Input: part model. Units: mm. Frame: model coordinates. Face numbers are marked on the shaded views. A direction names the side the tool comes from. Give positions to 0.01 mm unless a question says otherwise; leave off trailing zeros. Loops run counter-clockwise (first coordinate to the right, second up) from the corner with the lowest first, then second, coordinate; pieces in that order, holes last.
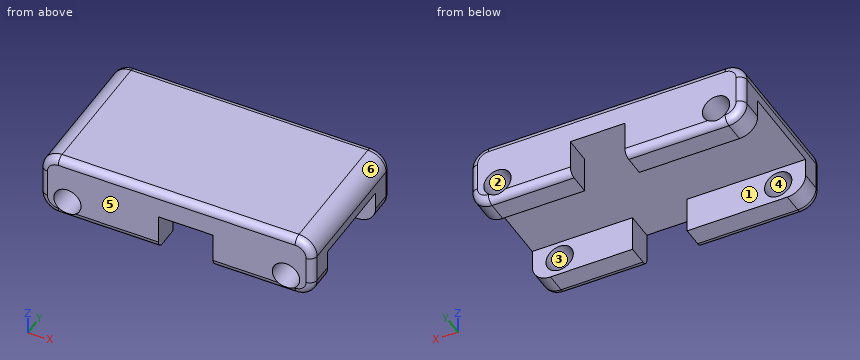
from build123d import *

# Parameters (mm, degrees)
F0_R          = 4.7625
F1_DEPTH      = 25.4
F2_W          = 31.75
F2_H          = 12.7
F3_DEPTH      = 47.626
F3_DEPTH_BACK = 47.626
F4_T1_DEPTH   = 82.55
F4_T3_DEPTH   = 9.6279704779
F4_T5_DEPTH   = 41.275
F4_T7_DEPTH   = 34.925
F4_T10_ANGLE  = 90
F4_T12_ANGLE  = 90
F4_T14_ANGLE  = 90
F4_T16_ANGLE  = 90
F4_T18_ANGLE  = 90
F4_T20_ANGLE  = 90
F4_T22_ANGLE  = 90
F4_T24_ANGLE  = 90


# Not quite as in the source:
# - a fillet or chamfer that OpenCascade refuses, or shapes differently, is made with other operations: its cross-section is extruded or revolved along the edge and cut away or added


with BuildPart() as f1:
    # F0 (on Front) → F1 (new body, symmetric)
    with BuildSketch(Plane.XZ):
        with BuildLine():
            Line((41.275, 15.9779704779), (-41.275, 15.9779704779))
            ThreePointArc((-41.275, 15.9779704779), (-45.7651280605, 14.1180985385), (-47.625, 9.6279704779))
            Line((-47.625, 9.6279704779), (-47.625, 0))
            ThreePointArc((-47.625, 0), (-45.7651280605, -4.4901280605), (-41.275, -6.35))
            Line((-41.275, -6.35), (-6.35, -6.35))
            Line((-6.35, -6.35), (-6.35, 6.35))
            Line((-6.35, 6.35), (12.7, 6.35))
            Line((12.7, 6.35), (12.7, -6.35))
            Line((12.7, -6.35), (41.275, -6.35))
            ThreePointArc((41.275, -6.35), (45.7651280605, -4.4901280605), (47.625, 0))
            Line((47.625, 0), (47.625, 9.6279704779))
            ThreePointArc((47.625, 9.6279704779), (45.7651280605, 14.1180985385), (41.275, 15.9779704779))
        make_face()
        with Locations((-38.1, 0)):
            Circle(F0_R, mode=Mode.SUBTRACT)
        with Locations((38.1, 0)):
            Circle(F0_R, mode=Mode.SUBTRACT)
    extrude(amount=F1_DEPTH, both=True)

    # F2 (on Right) → F3 (cut, two sides)
    with BuildSketch(Plane.YZ) as f3_sk:
        Rectangle(F2_W, F2_H)
    extrude(amount=F3_DEPTH, mode=Mode.SUBTRACT)
    extrude(f3_sk.sketch, amount=-F3_DEPTH_BACK, mode=Mode.SUBTRACT)

    # F4: fillet of radius 2.54 on 18 edges, made by hand

    # F4_s2 → F4_t1 (cut)
    with BuildSketch(Plane.YZ.offset(-41.275)):
        with BuildLine():
            ThreePointArc((22.86, 15.9779704779), (24.6560512242, 15.2340217022), (25.4, 13.4379704779))
            Line((25.4, 13.4379704779), (25.4, 15.9779704779))
            Line((25.4, 15.9779704779), (22.86, 15.9779704779))
        make_face()
        with BuildLine():
            ThreePointArc((-22.86, 15.9779704779), (-24.6560512242, 15.2340217022), (-25.4, 13.4379704779))
            Line((-25.4, 13.4379704779), (-25.4, 15.9779704779))
            Line((-25.4, 15.9779704779), (-22.86, 15.9779704779))
        make_face()
    extrude(amount=F4_T1_DEPTH, mode=Mode.SUBTRACT)

    # F4_s4 → F4_t3 (cut)
    with BuildSketch(Plane.XY):
        with BuildLine():
            ThreePointArc((-45.085, 25.4), (-46.8810512242, 24.6560512242), (-47.625, 22.86))
            Line((-47.625, 22.86), (-47.625, 25.4))
            Line((-47.625, 25.4), (-45.085, 25.4))
        make_face()
        with BuildLine():
            ThreePointArc((45.085, 25.4), (46.8810512242, 24.6560512242), (47.625, 22.86))
            Line((47.625, 22.86), (47.625, 25.4))
            Line((47.625, 25.4), (45.085, 25.4))
        make_face()
        with BuildLine():
            ThreePointArc((-45.085, -25.4), (-46.8810512242, -24.6560512242), (-47.625, -22.86))
            Line((-47.625, -22.86), (-47.625, -25.4))
            Line((-47.625, -25.4), (-45.085, -25.4))
        make_face()
        with BuildLine():
            ThreePointArc((45.085, -25.4), (46.8810512242, -24.6560512242), (47.625, -22.86))
            Line((47.625, -22.86), (47.625, -25.4))
            Line((47.625, -25.4), (45.085, -25.4))
        make_face()
    extrude(amount=F4_T3_DEPTH, mode=Mode.SUBTRACT)

    # F4_s6 → F4_t5 (cut)
    with BuildSketch(Plane.YZ.offset(-41.275)):
        with BuildLine():
            ThreePointArc((25.4, -3.81), (24.6560512242, -5.6060512242), (22.86, -6.35))
            Line((22.86, -6.35), (25.4, -6.35))
            Line((25.4, -6.35), (25.4, -3.81))
        make_face()
        with BuildLine():
            ThreePointArc((-25.4, -3.81), (-24.6560512242, -5.6060512242), (-22.86, -6.35))
            Line((-22.86, -6.35), (-25.4, -6.35))
            Line((-25.4, -6.35), (-25.4, -3.81))
        make_face()
    extrude(amount=F4_T5_DEPTH, mode=Mode.SUBTRACT)

    # F4_s8 → F4_t7 (cut)
    with BuildSketch(Plane.YZ.offset(6.35)):
        with BuildLine():
            ThreePointArc((25.4, -3.81), (24.6560512242, -5.6060512242), (22.86, -6.35))
            Line((22.86, -6.35), (25.4, -6.35))
            Line((25.4, -6.35), (25.4, -3.81))
        make_face()
        with BuildLine():
            ThreePointArc((-25.4, -3.81), (-24.6560512242, -5.6060512242), (-22.86, -6.35))
            Line((-22.86, -6.35), (-25.4, -6.35))
            Line((-25.4, -6.35), (-25.4, -3.81))
        make_face()
    extrude(amount=F4_T7_DEPTH, mode=Mode.SUBTRACT)

    # F4_s9 → F4_t10 (revolve, cut)
    with BuildSketch(Plane.YZ.offset(-41.275)):
        with BuildLine():
            ThreePointArc((25.4, 13.4379704779), (24.6560512242, 15.2340217022), (22.86, 15.9779704779))
            Line((22.86, 15.9779704779), (25.4, 15.9779704779))
            Line((25.4, 15.9779704779), (25.4, 13.4379704779))
        make_face()
    revolve(axis=Axis((-41.275, 25.4, 9.6279704779), (0, -1, 0)), revolution_arc=F4_T10_ANGLE, mode=Mode.SUBTRACT)

    # F4_s11 → F4_t12 (revolve, cut)
    with BuildSketch(Plane.XY):
        with BuildLine():
            ThreePointArc((-45.085, 25.4), (-46.8810512242, 24.6560512242), (-47.625, 22.86))
            Line((-47.625, 22.86), (-47.625, 25.4))
            Line((-47.625, 25.4), (-45.085, 25.4))
        make_face()
    revolve(axis=Axis((-41.275, 25.4, 0), (0, -1, 0)), revolution_arc=F4_T12_ANGLE, mode=Mode.SUBTRACT)

    # F4_s13 → F4_t14 (revolve, cut)
    with BuildSketch(Plane.YZ.offset(41.275)):
        with BuildLine():
            ThreePointArc((25.4, -3.81), (24.6560512242, -5.6060512242), (22.86, -6.35))
            Line((22.86, -6.35), (25.4, -6.35))
            Line((25.4, -6.35), (25.4, -3.81))
        make_face()
    revolve(axis=Axis((41.275, 25.4, 0), (0, -1, 0)), revolution_arc=F4_T14_ANGLE, mode=Mode.SUBTRACT)

    # F4_s15 → F4_t16 (revolve, cut)
    with BuildSketch(Plane.XY.offset(9.6279704779)):
        with BuildLine():
            ThreePointArc((45.085, 25.4), (46.8810512242, 24.6560512242), (47.625, 22.86))
            Line((47.625, 22.86), (47.625, 25.4))
            Line((47.625, 25.4), (45.085, 25.4))
        make_face()
    revolve(axis=Axis((41.275, 25.4, 9.6279704779), (0, -1, 0)), revolution_arc=F4_T16_ANGLE, mode=Mode.SUBTRACT)

    # F4_s17 → F4_t18 (revolve, cut)
    with BuildSketch(Plane.YZ.offset(-41.275)):
        with BuildLine():
            ThreePointArc((-22.86, 15.9779704779), (-24.6560512242, 15.2340217022), (-25.4, 13.4379704779))
            Line((-25.4, 13.4379704779), (-25.4, 15.9779704779))
            Line((-25.4, 15.9779704779), (-22.86, 15.9779704779))
        make_face()
    revolve(axis=Axis((-41.275, -25.4, 9.6279704779), (0, -1, 0)), revolution_arc=F4_T18_ANGLE, mode=Mode.SUBTRACT)

    # F4_s19 → F4_t20 (revolve, cut)
    with BuildSketch(Plane.XY):
        with BuildLine():
            ThreePointArc((-45.085, -25.4), (-46.8810512242, -24.6560512242), (-47.625, -22.86))
            Line((-47.625, -22.86), (-47.625, -25.4))
            Line((-47.625, -25.4), (-45.085, -25.4))
        make_face()
    revolve(axis=Axis((-41.275, -25.4, 0), (0, -1, 0)), revolution_arc=F4_T20_ANGLE, mode=Mode.SUBTRACT)

    # F4_s21 → F4_t22 (revolve, cut)
    with BuildSketch(Plane.YZ.offset(41.275)):
        with BuildLine():
            ThreePointArc((-25.4, -3.81), (-24.6560512242, -5.6060512242), (-22.86, -6.35))
            Line((-22.86, -6.35), (-25.4, -6.35))
            Line((-25.4, -6.35), (-25.4, -3.81))
        make_face()
    revolve(axis=Axis((41.275, -25.4, 0), (0, -1, 0)), revolution_arc=F4_T22_ANGLE, mode=Mode.SUBTRACT)

    # F4_s23 → F4_t24 (revolve, cut)
    with BuildSketch(Plane.XY.offset(9.6279704779)):
        with BuildLine():
            ThreePointArc((45.085, -25.4), (46.8810512242, -24.6560512242), (47.625, -22.86))
            Line((47.625, -22.86), (47.625, -25.4))
            Line((47.625, -25.4), (45.085, -25.4))
        make_face()
    revolve(axis=Axis((41.275, -25.4, 9.6279704779), (0, -1, 0)), revolution_arc=F4_T24_ANGLE, mode=Mode.SUBTRACT)


solid = f1.part
(1) Cut plane A-A (x = -24). Return the cut outline in (y, z) (3 decimals).
Values follow:
outline: (-25.4, -3.81) arc R2.54 ccw to (-22.86, -6.35) - (-15.875, -6.35) - (-15.875, 6.35) - (15.875, 6.35) - (15.875, -6.35) - (22.86, -6.35) arc R2.54 ccw to (25.4, -3.81) - (25.4, 13.438) arc R2.54 ccw to (22.86, 15.978) - (-22.86, 15.978) arc R2.54 ccw to (-25.4, 13.438) - close
(2) Pin query (flat end, axial travel): pin 1 Ø4 at (y, z) = (-12, 1) entering from -X; pin 2 Ø6 at (x, y) = (-25, 14.5) entering from -Z; pin 3 Ø4 at (y, z) = (18.5, -3.5) entering from -X; pin 4 Ø10 at (x, y) = (3.5, -2.5) entering from -Z. Return the tip coordinate at first contact, or that it passes through.
Values follow:
pin 1: passes through
pin 2: stops at z = -6.35
pin 3: stops at x = -47.45
pin 4: stops at z = 6.35
(3) Cut plane B-B (x = 38.1). Count the separate pieces of the cut face and the enclosed holes in it, and give its area (3 significant figures).
Values follow:
separate pieces: 3
enclosed holes: 0
area: 544 mm2
(4) Reachability of the marked faces 1 and 2 from +Z, -Z, +X, -X, +Y, -Y: full face, straight path, thin tool, end or side. Return the list, or none.
Values follow:
face 1: -Z, +X, -X
face 2: +Y, -Y
(5) Mould query, pull axis Z, two halves, no side actions, for the marked faces 3, 4, 5 and 6. Classes: +Z half, -Z half, draft (parallel to the pull), parting line (faces both ways), or undercut.
Values follow:
face 3: undercut
face 4: undercut
face 5: draft
face 6: +Z half
(6) Ray query, probe 1 along Z at (x, y) = (-38, -20); probe 2 along Y at (x, z) = (-24, -0.5) (3 decimals). Return the intervals inside material, ascending.
Values follow:
probe 1: z = -6.35 to -4.76, 4.76 to 15.98
probe 2: y = -25.4 to -15.875, 15.875 to 25.4
(7) Cut plane C-C (y = 0). Return the cut outline in (x, z) (3 decimals).
Values follow:
outline: (-47.625, 6.35) - (47.625, 6.35) - (47.625, 9.628) arc R6.35 ccw to (41.275, 15.978) - (-41.275, 15.978) arc R6.35 ccw to (-47.625, 9.628) - close
